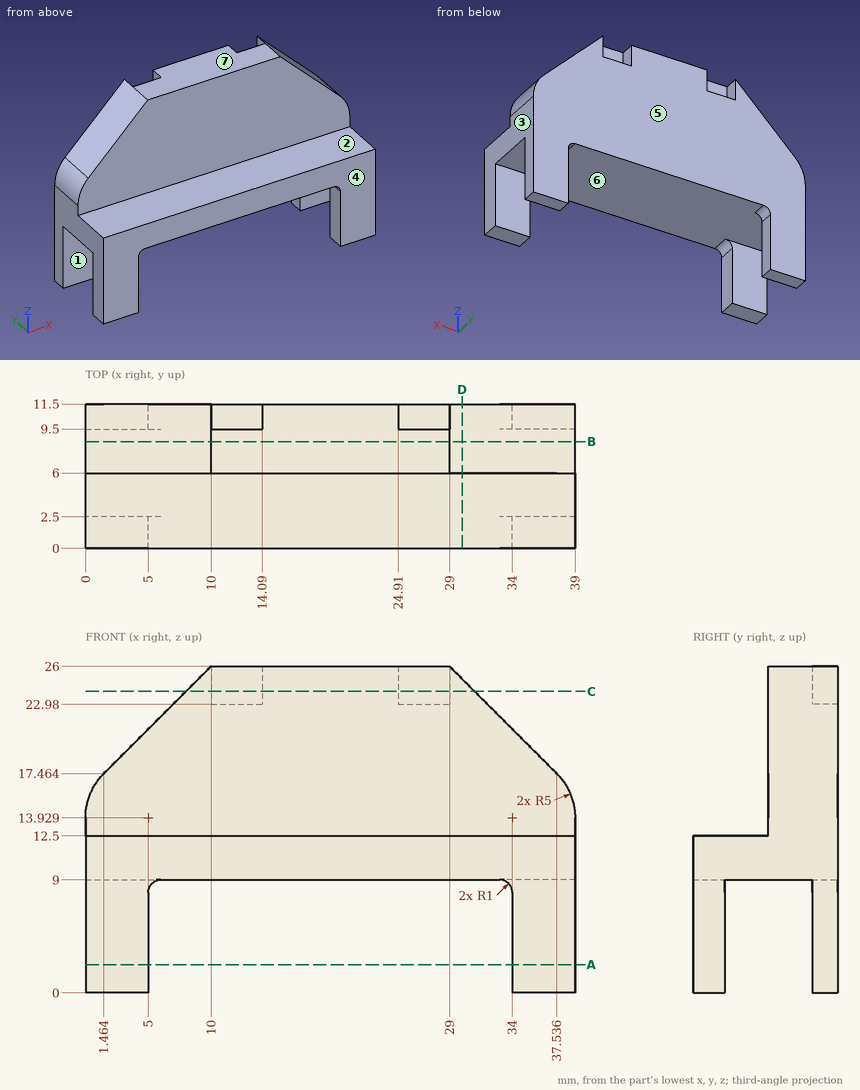
Study the drawing (mm; zero at the part's minimum x, y, z) and answer. A direction names the side the tool comes from. Coordinates: 2 decimals unless noted, no trailing zeros. Write each loop counter-clockwise with the first axis right and the second up, starting at its lowest first coordinate (ties: lowest second). Pieces come first, ordered by that corner, then holes. Notation, with made-up numbers: M 70,76 L 94,76 A23 ccw 94,93 Z; hole C 66,-4.5 d5. An arc over 180 degrees is marked long. Use a Markdown table: item, result. Add a question column.
1. Section C-C (z = 24) is taken. Give the vertices of the cut face in (x, y).
2. Section B-B (y = 8.5) is taken. Give the vertices of the cut face in (x, z) (1 decimal).
3. Which of the six approach directions +Z, -Z, +X, -X, +Y, -Y give full straight-line access (tool end or side, diameter ignored) to the marked faces 1, 2 and 3?
4. Straight lines are drawn through the part: line 1 along Z through (x, y) = (13, 10.5); line 2 along Z through (x, y) = (24, 0.75); line 3 along Y through (x, z) = (37, 13.5). For each, find the intervals that lie inside material, in ascending order. Write a range as [from, to].
5. For a pull along Y with two mould halves and no side action, classify the marked faces 4, 5, 6 and 7 as +Y half, -Y half, draft (parallel to the pull), parting line (faces both ways), or undercut.
6. Section D-D (x = 30) is taken. Give the vertices of the cut face in (y, z), plus the area to 3 significant figures.
7. Given P1, Ø7, axis at x = 15.5, z = 18, coming from the -Y side; P2, Ø3.5, axis at x = 13, y = 5.5, coming from the -Z side; P3, Ø0.6, axis at y = 11, z = 25, coming from the +X side, each flat-ended and moving along its own axis, determine where each tip first touches the part or whether it passes through.
8. Section A-A (z = 2.25) is taken. Give the vertices of the cut face in (x, y).
Data:
| question | item | result |
|---|---|---|
| 1 | outline | M 8,6 L 31,6 L 31,11.5 L 29,11.5 L 29,9.5 L 24.91,9.5 L 24.91,11.5 L 14.09,11.5 L 14.09,9.5 L 10,9.5 L 10,11.5 L 8,11.5 Z |
| 2 | outline | M 0,9 L 39,9 L 39,13.9 A5 ccw 37.5,17.5 L 29,26 L 10,26 L 1.5,17.5 A5 ccw 0,13.9 Z |
| 3 | face 1 | -Z, +X, -X |
| 3 | face 2 | +Z, +X, -X, -Y |
| 3 | face 3 | +Z, -Z, +X, +Y, -Y |
| 4 | line 1 | z = [9, 22.98] |
| 4 | line 2 | z = [9, 12.5] |
| 4 | line 3 | y = [6, 11.5] |
| 5 | face 4 | -Y half |
| 5 | face 5 | +Y half |
| 5 | face 6 | undercut |
| 5 | face 7 | draft |
| 6 | outline | M 0,9 L 11.5,9 L 11.5,25 L 6,25 L 6,12.5 L 0,12.5 Z |
| 6 | area | 109 mm2 |
| 7 | P1 | stops at y = 6 |
| 7 | P2 | stops at z = 9 |
| 7 | P3 | stops at x = 30.3 |
| 8 | outline | M 0,0 L 5,0 L 5,2.5 L 0,2.5 Z; M 0,9.5 L 5,9.5 L 5,11.5 L 0,11.5 Z; M 34,0 L 39,0 L 39,2.5 L 34,2.5 Z; M 34,9.5 L 39,9.5 L 39,11.5 L 34,11.5 Z |
